from build123d import *

# Parameters (mm, degrees)
SKETCH1_W                = 353
SKETCH1_H                = 91
BOSS_EXTRUDE1_DEPTH      = 18
FILLET1_R                = 10
SKETCH3_OUTSIDE_W        = 427.996
SKETCH3_OUTSIDE_H        = 165.996
CUT_EXTRUDE1_DEPTH       = 12
CUT_EXTRUDE2_DEPTH       = 11
SKETCH5_R                = 6.5
BOSS_EXTRUDE2_DEPTH      = 1.5
CUT_EXTRUDE3_REACH       = 185.157
SKETCH8_W                = 80
SKETCH8_H                = 36
FILLET2_R                = 5
F_6_0_6_DIAMETER_HOLE1_D = 6
M5X0_8_TAPPED_HOLE1_D    = 4.2
M6X1_0_TAPPED_HOLE1_D    = 5
M3X0_5_TAPPED_HOLE1_D    = 2.5


with BuildPart() as part:
    # Sketch1 → Boss-Extrude1 (new body)
    with BuildSketch(Plane(origin=(0, 0, 0), x_dir=(1, 0, 0), z_dir=(0, 1, 0))):
        Rectangle(SKETCH1_W, SKETCH1_H)
    extrude(amount=BOSS_EXTRUDE1_DEPTH)

    # Fillet1
    fillet1_edges = [part.edges().sort_by_distance(p)[0] for p in [
        (-176.5, 9, -45.5),
        (176.5, 9, -45.5),
        (176.5, 9, 45.5),
        (-176.5, 9, 45.5),
    ]]
    fillet(fillet1_edges, radius=FILLET1_R)

    # Sketch3 outside → Cut-Extrude1 (cut)
    with BuildSketch(Plane(origin=(0, 18, 0), x_dir=(1, 0, 0), z_dir=(0, 1, 0))):
        Rectangle(SKETCH3_OUTSIDE_W, SKETCH3_OUTSIDE_H)
        with BuildLine():
            Line((-175, 35.5), (-175, -35.5))
            ThreePointArc((-175, -35.5), (-172.51040764, -41.51040764), (-166.5, -44))
            Line((-166.5, -44), (166.5, -44))
            ThreePointArc((166.5, -44), (172.51040764, -41.51040764), (175, -35.5))
            Line((175, -35.5), (175, 35.5))
            ThreePointArc((175, 35.5), (172.51040764, 41.51040764), (166.5, 44))
            Line((166.5, 44), (-166.5, 44))
            ThreePointArc((-166.5, 44), (-172.51040764, 41.51040764), (-175, 35.5))
        make_face(mode=Mode.SUBTRACT)
    extrude(amount=-CUT_EXTRUDE1_DEPTH, mode=Mode.SUBTRACT)

    # Sketch4 → Cut-Extrude2 (cut)
    with BuildSketch(Plane.XZ):
        with BuildLine():
            Line((-170, 35.5), (-170, -35.5))
            ThreePointArc((-170, -35.5), (-168.974873734, -37.974873734), (-166.5, -39))
            Line((-166.5, -39), (166.5, -39))
            ThreePointArc((166.5, -39), (168.974873734, -37.974873734), (170, -35.5))
            Line((170, -35.5), (170, 35.5))
            ThreePointArc((170, 35.5), (168.974873734, 37.974873734), (166.5, 39))
            Line((166.5, 39), (-166.5, 39))
            ThreePointArc((-166.5, 39), (-168.974873734, 37.974873734), (-170, 35.5))
        make_face()
    extrude(amount=-CUT_EXTRUDE2_DEPTH, mode=Mode.SUBTRACT)

    # Sketch5 → Boss-Extrude2 (add)
    with BuildSketch(Plane(origin=(0, 18, 0), x_dir=(1, 0, 0), z_dir=(0, 1, 0))):
        with Locations(Location((-166, 35, 0), (0, 0, 270))):
            Circle(SKETCH5_R)
        with Locations(Location((-166, -35, 0), (0, 0, 270))):
            Circle(SKETCH5_R)
        with Locations(Location((0, 35, 0), (0, 0, 270))):
            Circle(SKETCH5_R)
        with Locations(Location((0, -35, 0), (0, 0, 270))):
            Circle(SKETCH5_R)
        with Locations(Location((166, 35, 0), (0, 0, 270))):
            Circle(SKETCH5_R)
        with Locations(Location((166, -35, 0), (0, 0, 270))):
            Circle(SKETCH5_R)
    extrude(amount=BOSS_EXTRUDE2_DEPTH)

    # Sketch8 → Cut-Extrude3 (cut, up to next)
    with BuildSketch(Plane(origin=(0, 18, 0), x_dir=(1, 0, 0), z_dir=(0, 1, 0)), mode=Mode.PRIVATE) as cut_extrude3_sk1:
        with Locations((-122, 0)):
            Rectangle(SKETCH8_W, SKETCH8_H)
    cut_extrude3_tool1 = extrude(cut_extrude3_sk1.sketch, amount=-CUT_EXTRUDE3_REACH, mode=Mode.PRIVATE) & part.part
    add(cut_extrude3_tool1.solids().sort_by_distance((-122, 18, 0))[0], mode=Mode.SUBTRACT)

    # Fillet2
    fillet2_edges = [part.edges().sort_by_distance(p)[0] for p in [
        (-162, 14.5, 18),
        (-162, 14.5, -18),
        (-82, 14.5, -18),
        (-82, 14.5, 18),
    ]]
    fillet(fillet2_edges, radius=FILLET2_R)

    # Ø6.0 (6) Diameter Hole1 (through all)
    with Locations(Plane(origin=(0, 19.5, 0), x_dir=(1, 0, 0), z_dir=(0, 1, 0))):
        with Locations((-166, -35), (-166, 35), (0, 35), (0, -35), (166, 35), (166, -35)):
            Hole(F_6_0_6_DIAMETER_HOLE1_D / 2)

    # M5x0.8 Tapped Hole1 (through all)
    with Locations(Plane(origin=(0, 18, 0), x_dir=(1, 0, 0), z_dir=(0, 1, 0))):
        with Locations((-34, 35), (-16, 35), (40, 35), (58, 35), (-59, 15), (-59, -15), (93, -23), (145, -23), (145, 23), (93, 23)):
            Hole(M5X0_8_TAPPED_HOLE1_D / 2)

    # M6x1.0 Tapped Hole1 (through all)
    with Locations(Plane(origin=(0, 18, 0), x_dir=(1, 0, 0), z_dir=(0, 1, 0))):
        with Locations((-142, 25), (-97, 25)):
            Hole(M6X1_0_TAPPED_HOLE1_D / 2)

    # M3x0.5 Tapped Hole1 (through all)
    with Locations(Plane(origin=(0, 18, 0), x_dir=(1, 0, 0), z_dir=(0, 1, 0))):
        with Locations((29, -33), (69, -33), (69, -19), (29, -19)):
            Hole(M3X0_5_TAPPED_HOLE1_D / 2)


solid = part.part
Could you check a few things on this model? Use its own coordinates, in mm. A direction names the side the tool comes from. Give positions to 0.01 mm unless a question says otherwise; leave off trailing zeros. Order: outer loops, then holes, each group sorted by start corner. A loop starts at its lowest first (then second) coordinate and runs counter-clockwise, first axis right, second up.
1. I need wall thicknesses on L1, parallel to X at y = 14, z = 35; L2, parallel to X at y = 16.5, z = 23; L3, parallel to Z at x = -97, y = 15.5. Which ranges of each line are inside material? Lowest first, please.
Answers below:
L1: x = -175 to -169, -163 to -3, 3 to 163, 169 to 175
L2: x = -175 to 90.9, 95.1 to 142.9, 147.1 to 175
L3: z = -44 to -27.5, -22.5 to -18, 18 to 44
2. Suppose I cut it at D-D (x = 110). Write out the boundary of the cut face in (y, z), plus the area to 3 significant figures.
Answers below:
outline: (0, -45.5) - (6, -45.5) - (6, -44) - (18, -44) - (18, 44) - (6, 44) - (6, 45.5) - (0, 45.5) - (0, 39) - (11, 39) - (11, -39) - (0, -39) - close
area: 744 mm2
3. Suppose I cut it at B-B (x = -122.5). Write out the boundary of the cut face in (y, z).
Answers below:
outline: (0, -45.5) - (6, -45.5) - (6, -44) - (18, -44) - (18, -18) - (11, -18) - (11, -39) - (0, -39) - close; (0, 39) - (11, 39) - (11, 18) - (18, 18) - (18, 44) - (6, 44) - (6, 45.5) - (0, 45.5) - close
4. Suppose I cut it at A-A (z = -1.5). Write out the boundary of the cut face in (x, y).
Answers below:
outline: (-176.5, 0) - (-170, 0) - (-170, 11) - (-162, 11) - (-162, 18) - (-175, 18) - (-175, 6) - (-176.5, 6) - close; (-82, 11) - (170, 11) - (170, 0) - (176.5, 0) - (176.5, 6) - (175, 6) - (175, 18) - (-82, 18) - close
5. For pin 1 (5 mm diameter, centred on x = 145, z = -23, fed in from +Y); pin 2 (6 mm diameter, centred on x = -33, y = 17.5, fed in from +Z); pin 3 (9.5 mm diameter, centred on x = 166, z = 35, fed in from +Y); pin 4 (7.5 mm diameter, centred on x = -133.5, y = 15.5, fed in from -Z), each with a flat end and sliding along its axis, tell me the tip position at first contact or that it passes through.
Answers below:
pin 1: stops at y = 18
pin 2: stops at z = 44
pin 3: stops at y = 19.5
pin 4: stops at z = -44
6. Which directions (+Z, -Z, +X, -X, +Y, -Y) give clear straight access to the entire face, cutting with the end or side of a thin tool? Please do faces 1 (the flat face through (-162, 15, 0)), 2 (the flat face through (175, 12, 0)), 3 (the flat face through (-2, 12, 44)), 4 (the flat face through (35, 11, 1)), 5 (the cylindrical face through (-172.345, 18.74, 33.591)).
Answers below:
face 1: +Y, -Y
face 2: +Z, -Z, +X, +Y
face 3: +Z, +X, -X, +Y
face 4: -Y
face 5: +Y
7. Suppose I cut it at C-C (x = 0). Write out the boundary of the cut face in (y, z), plus the area to 3 significant figures.
Answers below:
outline: (0, -45.5) - (6, -45.5) - (6, -44) - (18, -44) - (18, -41.5) - (19.5, -41.5) - (19.5, -38) - (11, -38) - (11, -39) - (0, -39) - close; (0, 39) - (11, 39) - (11, 38) - (19.5, 38) - (19.5, 41.5) - (18, 41.5) - (18, 44) - (6, 44) - (6, 45.5) - (0, 45.5) - close; (11, -32) - (19.5, -32) - (19.5, -28.5) - (18, -28.5) - (18, 28.5) - (19.5, 28.5) - (19.5, 32) - (11, 32) - close
area: 681 mm2
